Could you check a few things on this model? Use its own coordinates, in mm. Give positions to 0.01 mm unless a question says otherwise; leave off trailing zeros. Order: outer loops, then holes, each group sorted by start corner. A loop starts at its lowest first (then second) coordinate and runs counter-clockwise, first axis right, second up. Notation, with made-up numbers: (-10, 40) - (14, 40) arc R22 cw to (14, 70) - close; hole circle Ø8 at (-8.75, -39.5). An arc over 180 degrees is marked (long way). Put each result on its own line as item: value.
Autodesk Inventor part; units mm, degrees
ref_plane "YZ Plane" through (0, 0, 0) normal (1, 0, 0) x (0, 1, 0)
ref_plane "XZ Plane" through (0, 0, 0) normal (0, 1, 0) x (-1, 0, 0)
ref_plane "XY Plane" through (0, 0, 0) normal (0, 0, 1) x (1, 0, 0)
sketch "Sketch2" plane through (0, 0, 0) normal (0, 1, 0) x (-1, 0, 0)
  line L0 (1.35, 0) -> (1.35, -4.5)
  line L1 (-1.35, -1) -> (-1.35, 3)
  line L2 (-1.35, -4.5) -> (-1.35, 3)
  line L3 (-1.35, 3) -> (1.35, 3)
  line L4 (1.35, 3) -> (1.35, -4.5)
  line L5 (-1.35, -4.5) -> (1.35, -4.5)
  point P0 (0, 0)
  dimension "d8" = 1.35
  dimension "d11" = 4
  dimension "d24" = 7.5
  dimension "d62" = 2.7
  dimension "d63" = 2.7
extrude "Extrusion1" add sketch "Sketch2" along normal mid plane 2
sketch "Sketch6" plane through (0, 1, 0) normal (0, 1, 0) x (1, 0, 0)
  line L0 (0, -3) -> (0, -1)
  circle A0 centre (0, -1) radius 0.8
  line L1 (0, -1) -> (-1.35, -1)
  line L2 (-1.35, 4.5) -> (-1.35, -3)
  point P0 (0, 0)
  dimension "d40" = 2
  dimension "d41" = 1.6
  dimension "d64" = 1.35
hole "Hole3" at (0, 1, 1) direction (0, -1, 0) diameter 1.6 end through all
sketch "Sketch7" plane through (0, 1, 0) normal (0, 1, 0) x (1, 0, 0)
  line L0 (0, 4.5) -> (0, 3.5)
  circle A0 centre (0, 3.5) radius 0.5
  line L1 (0, 3.5) -> (0, -1)
  line L2 (0, 3.5) -> (0, 1)
  line L3 (0, 4.5) -> (0, 4)
  point P0 (0, 0)
  dimension "d50" = 1
  dimension "d49" = 1
  dimension "d51" = 4.5
  dimension "d52" = 2.5
  dimension "d53" = 0.5
hole "Hole4" at (0, 1, -3.5) direction (0, -1, 0) diameter 1 end through all
properties part number "Part3_slider" material "ABS Plastic"
1) If I drill on line 1 (Z direction, x = 0, y = -0.15); line 2 (X direction, y = 0.2, z = -3.5); line 3 (Z direction, x = 0.35, y = 0.1), over which ranges is the centre line in solid material (lowest first)? Write a range as [from, to].
Filled in:
line 1: z = [-4.5, -4], [-3, 0.2], [1.8, 3]
line 2: x = [-1.35, -0.5], [0.5, 1.35]
line 3: z = [-4.5, -3.86], [-3.14, 0.28], [1.72, 3]
2) We'd pull the mould along Z, two halves only. Please class faces 1 (the flat face through (0, 0, 3)), 2 (the flat face through (-1.35, 0, -1)), 3 (the cylindrical face through (0, 0, -4)): pulls with the +Z half, pulls with the -Z half, needs draft (parallel to the pull), parting line crosses it, or undercut.
Filled in:
face 1: pulls with the +Z half
face 2: needs draft
face 3: undercut
3) Suppose I cut it at B-B, the plane z = 1.5. List the corners of the cut face in (x, y) for me, and give its area (3 significant figures).
Filled in:
outline: (-1.35, -1) - (-0.62, -1) - (-0.62, 1) - (-1.35, 1) - close; (0.62, -1) - (1.35, -1) - (1.35, 1) - (0.62, 1) - close
area: 2.90 mm^2
4) I'm going to push a flat-ended pin straight in: pin 1 (1 mm diameter, centred on x = 0, z = 1, fed in from -Y). Where does the tip first touch, or does it pass through?
Filled in:
pin 1: passes through
5) Suppose I cut it at A-A, the plane x = 0. List the corners of the cut face in (y, z) for me, and give its area (3 significant figures).
Filled in:
outline: (-1, -4.5) - (1, -4.5) - (1, -4) - (-1, -4) - close; (-1, -3) - (1, -3) - (1, 0.2) - (-1, 0.2) - close; (-1, 1.8) - (1, 1.8) - (1, 3) - (-1, 3) - close
area: 9.80 mm^2
6) Suppose I cut it at C-C, the plane x = 0.65. List the corners of the cut face in (y, z) for me.
Filled in:
outline: (-1, -4.5) - (1, -4.5) - (1, 0.53) - (-1, 0.53) - close; (-1, 1.47) - (1, 1.47) - (1, 3) - (-1, 3) - close
